Input: part model. Units: mm. Frame: model coordinates. A direction names the side the tool comes from. Round coordinates to 2 decimals unless told otherwise and drop trailing zeros. Write each loop counter-clockwise with the first axis right and the second up, starting at its lowest first coordinate (ties: lowest second). Pieces come first, ordered by that corner, then holes. Notation, with made-up numbers: (-21.75, -4.5) -> (17.25, -4.5) arc R26 ccw to (17.25, 15.5) -> close; hole circle Ø6 at (80.25, -29). An arc over 180 degrees is marked (long way). Use CSV: the item, a comma, the result in double quotes.
```python
from build123d import *

# Parameters (mm, degrees)
SKETCH_1_W            = 5
SKETCH_1_H            = 5
EXTRUDE_1_DEPTH       = 38.1
SKETCH_3_W            = 2
SKETCH_3_H            = 2.78
EXTRUDE_2_DEPTH       = 38.1
SKETCH_6_W            = 5
SKETCH_6_H            = 5
SKETCH_6_W_2          = 4.4
SKETCH_6_H_2          = 4.4
CUT_EXTRUDE_1_DEPTH   = 39.545277272
EXTRUDE_3_DEPTH       = 38.1
SKETCH_9_W            = 0.05
SKETCH_9_H            = 2.78
CUT_EXTRUDE_1_2_DEPTH = 39.526982752
SKETCH_11_W           = 0.05
SKETCH_11_H           = 2.78
CUT_EXTRUDE_2_DEPTH   = 39.526982752


with BuildPart() as part:
    # Sketch 1 → Extrude 1 (new body)
    with BuildSketch(Plane(origin=(0, 0, 0), x_dir=(1, 0, 0), z_dir=(0, 1, 0))):
        Rectangle(SKETCH_1_W, SKETCH_1_H)
    extrude(amount=EXTRUDE_1_DEPTH)

    # Sketch 3 → Extrude 2 (add)
    with BuildSketch(Plane(origin=(0, 38.1, 0), x_dir=(1, 0, 0), z_dir=(0, 1, 0))):
        with Locations((0, -3.89)):
            Rectangle(SKETCH_3_W, SKETCH_3_H)
    extrude(amount=-EXTRUDE_2_DEPTH)

    # Sketch 6 → Cut-Extrude 1 (cut, through all)
    with BuildSketch(Plane.XZ):
        Rectangle(SKETCH_6_W, SKETCH_6_H)
        Rectangle(SKETCH_6_W_2, SKETCH_6_H_2, mode=Mode.SUBTRACT)
    extrude(amount=-CUT_EXTRUDE_1_DEPTH, mode=Mode.SUBTRACT)


with BuildPart() as cut_extrude_1_piece_1:
    # of the separate pieces the step leaves, piece 1, a body of its own (cut_extrude_1_pieces)
    add(part.part.solids().sort_by_distance((2.2, 0, 2.2))[0])



with BuildPart() as cut_extrude_1_piece_2:
    # of the separate pieces the step leaves, piece 2, a body of its own (cut_extrude_1_pieces)
    add(part.part.solids().sort_by_distance((-1, 0, 5.28))[0])


with BuildPart() as cut_extrude_1_piece_1_1:
    add(cut_extrude_1_piece_1.part)

    add(cut_extrude_1_piece_2.part)  # Extrude 3 merges Cut-Extrude 1 piece 2
    # Sketch 8 → Extrude 3 (add)
    with BuildSketch(Plane.XZ):
        Polygon((1, 2.5), (2.2, 2.5), (2.2, 2.2), (-2.2, 2.2), (-2.2, 2.5), align=None)
    extrude(amount=-EXTRUDE_3_DEPTH)

    # Sketch 9 → Cut-Extrude 1 2 (cut, through all)
    with BuildSketch(Plane.XZ):
        with Locations((-0.975, 3.89)):
            Rectangle(SKETCH_9_W, SKETCH_9_H)
    extrude(amount=-CUT_EXTRUDE_1_2_DEPTH, mode=Mode.SUBTRACT)

    # Sketch 11 → Cut-Extrude 2 (cut, through all)
    with BuildSketch(Plane.XZ):
        with Locations((0.975, 3.89)):
            Rectangle(SKETCH_11_W, SKETCH_11_H)
    extrude(amount=-CUT_EXTRUDE_2_DEPTH, mode=Mode.SUBTRACT)


solid = cut_extrude_1_piece_1_1.part
```
Item 1: Section query C-C on z = 3. Return the cut outline in (x, y).
Worked answers:
outline,"(-0.95, 0) -> (0.95, 0) -> (0.95, 38.1) -> (-0.95, 38.1) -> close"
Item 2: Section query A-A on y = 33.5. Return the cut outline in (x, z).
Worked answers:
outline,"(-2.2, -2.2) -> (2.2, -2.2) -> (2.2, 2.5) -> (0.95, 2.5) -> (0.95, 5.28) -> (-0.95, 5.28) -> (-0.95, 2.5) -> (-2.2, 2.5) -> close"
Item 3: Line query: line 1 (X direction, y = 30, z = 4.25); line 2 (Z direction, x = -1.15, y = 31.5). Output: solid intervals per line, ascending.
Worked answers:
line 1,"x = -0.95 to 0.95"
line 2,"z = -2.2 to 2.5"
Item 4: Set-up query: faces 1 (the face through (2, 19, 2.5)), 2 (the face through (-0.95, 19, 4)), 3 (the face through (2.2, 19, 0)). Return all of +Z, -Z, +X, -X, +Y, -Y with unobstructed straight access to the full face (end or side cutting, diameter ignored); none if empty.
Worked answers:
face 1,"+Z, +X, +Y, -Y"
face 2,"+Z, -X, +Y, -Y"
face 3,"+Z, -Z, +X, +Y, -Y"
Item 5: Section query B-B on x = 1.6. Return the cut outline in (y, z), plus the area to 3 significant figures.
Worked answers:
outline,"(0, -2.2) -> (38.1, -2.2) -> (38.1, 2.5) -> (0, 2.5) -> close"
area,"179 mm²"
Item 6: First-contact query: pin 1 Ø1.4 at (y, z) = (19, 4.5) entering from -X; pin 2 Ø0.6 at (x, y) = (2, 19) entering from +Z; pin 3 Ø0.8 at (y, z) = (25.5, 3.5) entering from +X; pin 4 Ø2 at (x, y) = (1.5, 26) entering from +Z. Flat tips, straight axial feed; report the tip coordinate or a pass-through.
Worked answers:
pin 1,"stops at x = -0.95"
pin 2,"stops at z = 2.5"
pin 3,"stops at x = 0.95"
pin 4,"stops at z = 5.28"
